Drawing for the job (mm, zero at the part's lowest x, y, z). Coordinates: 2 decimals unless noted, no trailing zeros. Write each loop counter-clockwise with the first axis right and the second up, starting at its lowest first coordinate (ties: lowest second). Pieces come first, ordered by that corner, then holes. Notation, with made-up numbers: M 77.25,18 L 120.25,18 A12 cw 120.25,22 Z; hole C -39,-9 d9. An arc over 180 degrees is marked long. Put each result on its own line as item: value. Start each with the question number.
Q1. Cut at B-B (x = 1). Write the cut outline in (y, z).
Q2. Drill centre lines: line 1 along Y through (x, z) = (5, 2.5); line 2 along Y through (x, z) = (4, 8.5); line 3 along X through (y, z) = (1.55, 7.75). Where is each one in solid material? Low to high.
Q3. Drop flat-ended pins along their axis: pin 1 (5 mm diameter, centred on x = 3.5, z = 2.5, fed in from -Y); pin 2 (2 mm diameter, centred on x = 6.5, y = 1, fed in from -Z); pin 3 (3 mm diameter, centred on x = 7.5, z = 9.5, fed in from -Y); pin 4 (1.5 mm diameter, centred on x = 2, y = 1, fed in from -Z). Give the stop position or say it passes through.
Q4. Cut at A-A (y = 4.4). Write the cut outline in (x, z).
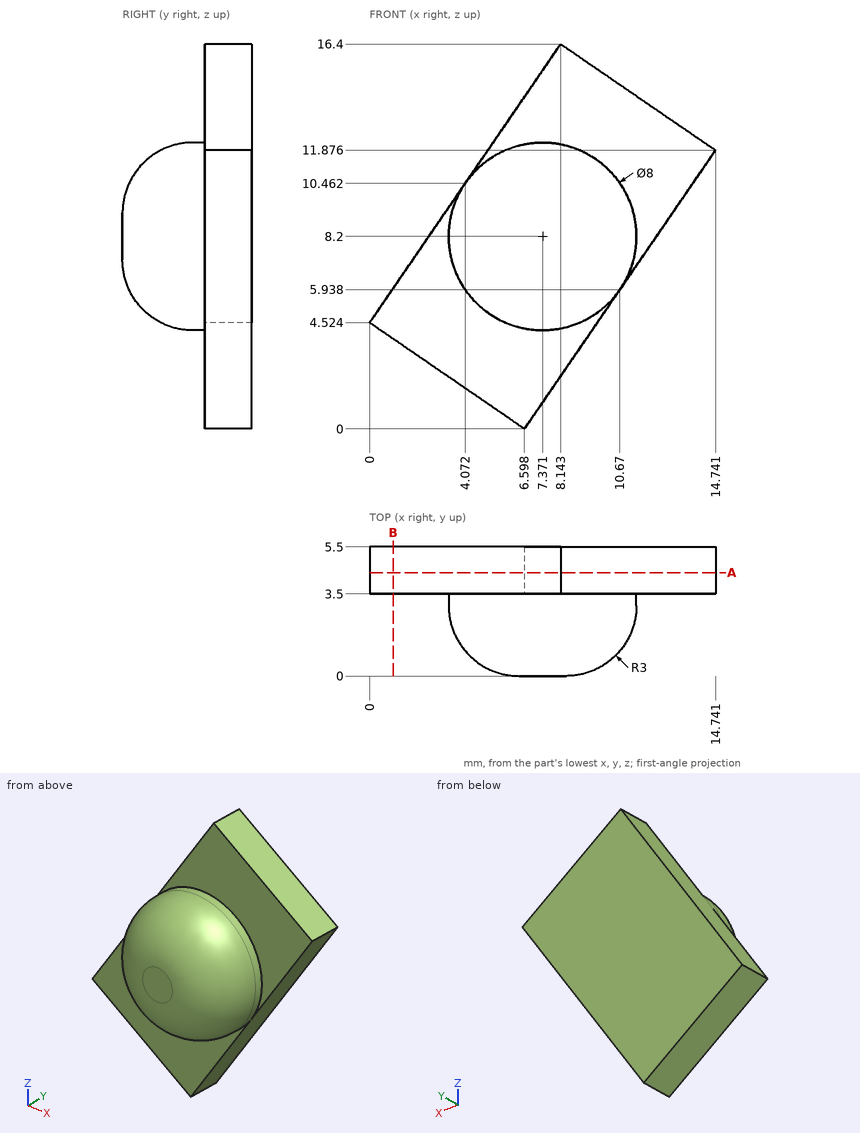
Computed values:
1. outline: M 3.5,3.84 L 5.5,3.84 L 5.5,5.98 L 3.5,5.98 Z
2. line 1: 3.5 to 5.5
2. line 2: 1.18 to 5.5
2. line 3: 3.77 to 10.97
3. pin 1: y = 3.5
3. pin 2: z = 4.43
3. pin 3: y = 0
3. pin 4: through
4. outline: M 0,4.52 L 6.6,0 L 14.74,11.88 L 8.14,16.4 Z
